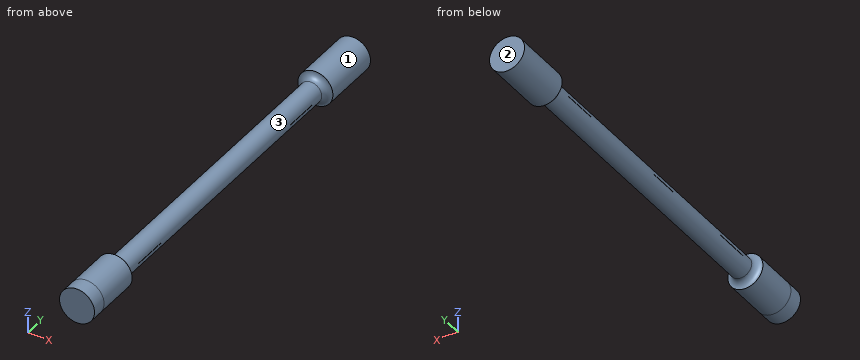
from build123d import *

# Parameters (mm, degrees)
SKETCH1_R               = 21.39
BOSS_EXTRUDE1_DEPTH     = 630
SKETCH2_R               = 35
BOSS_EXTRUDE2_DEPTH     = 88.02
BOSS_EXTRUDE3_START     = 88.02
SKETCH3_R               = 35
BOSS_EXTRUDE3_DEPTH     = 88.02
FILLET3_R               = 13.575
MOVE_FACE1_BY           = 30
MOVE_FACE2_BY           = 30
CUT_EXTRUDE1_DEPTH      = 750.655867982
CUT_EXTRUDE1_DEPTH_BACK = 750.655867982
CUT_EXTRUDE2_START      = -21.390000045
CUT_EXTRUDE2_DEPTH      = 21.390000045


# Read off the part's stored shape, not the designer's step: Cut-Extrude2
with BuildPart() as part:
    # Sketch1 → Boss-Extrude1 (new body)
    with BuildSketch(Plane(origin=(0, 0, 0), x_dir=(1, 0, 0), z_dir=(0, 1, 0))):
        with Locations(Location((0, 0, 0), (0, 0, 270))):
            Circle(SKETCH1_R)
    extrude(amount=BOSS_EXTRUDE1_DEPTH)

    # Sketch2 → Boss-Extrude2 (add)
    with BuildSketch(Plane(origin=(0, 630, 0), x_dir=(1, 0, 0), z_dir=(0, 1, 0))):
        with Locations(Location((0, 0, 0), (0, 0, 270))):
            Circle(SKETCH2_R)
    extrude(amount=BOSS_EXTRUDE2_DEPTH)

    # Sketch3 → Boss-Extrude3 (add)
    with BuildSketch(Plane.XZ.offset(BOSS_EXTRUDE3_START)):
        with Locations(Location((0, 0, 0), (0, 0, 90))):
            Circle(SKETCH3_R)
    extrude(amount=-BOSS_EXTRUDE3_DEPTH)

    # Fillet3
    fillet3_edges = [part.edges().sort_by_distance(p)[0] for p in [
        (0, 630, -21.39),
        (0, 0, -21.39),
    ]]
    fillet(fillet3_edges, radius=FILLET3_R)

    # Move Face1: a face moved outward by 30.0
    extrude(part.faces().sort_by_distance((0, 718.02, 0))[0], amount=MOVE_FACE1_BY, dir=(0, 1, 0))

    # Move Face2: a face moved outward by 30.0
    extrude(part.faces().sort_by_distance((0, -88.02, 0))[0], amount=MOVE_FACE2_BY, dir=(0, -1, 0))

    # Sketch4 → Cut-Extrude1 (cut, two sides: drawn at the far end of the back side and taken through both)
    with BuildSketch(Plane(origin=(0, 0, 0), x_dir=(0, 0, -1), z_dir=(1, 0, 0)).offset(-CUT_EXTRUDE1_DEPTH_BACK)):
        with BuildLine():
            Line((-0.43, 588.175), (-0.43, 518.175))
            ThreePointArc((-0.43, 518.175), (0, 517.745), (0.43, 518.175))
            Line((0.43, 518.175), (0.43, 588.175))
            ThreePointArc((0.43, 588.175), (0, 588.605), (-0.43, 588.175))
        make_face()
        with BuildLine():
            Line((-0.43, 111.71612329), (-0.43, 41.71612329))
            ThreePointArc((-0.43, 41.71612329), (0, 41.28612329), (0.43, 41.71612329))
            Line((0.43, 41.71612329), (0.43, 111.71612329))
            ThreePointArc((0.43, 111.71612329), (0, 112.14612329), (-0.43, 111.71612329))
        make_face()
    extrude(amount=CUT_EXTRUDE1_DEPTH + CUT_EXTRUDE1_DEPTH_BACK, mode=Mode.SUBTRACT)

    # Cut-Extrude2 outline → Cut-Extrude2 (cut)
    with BuildSketch(Plane(origin=(0, 0, 0), x_dir=(0, 0, -1), z_dir=(1, 0, 0)).offset(CUT_EXTRUDE2_START)):
        with BuildLine():
            ThreePointArc((-0.43, 260.7089), (0, 260.2789), (0.43, 260.7089))
            Line((0.43, 260.7089), (0.43, 320.7089))
            ThreePointArc((0.43, 320.7089), (0, 321.1389), (-0.43, 320.7089))
            Line((-0.43, 320.7089), (-0.43, 260.7089))
        make_face()
    extrude(amount=CUT_EXTRUDE2_DEPTH, mode=Mode.SUBTRACT)


solid = part.part
Can you work these out from the model? Positions are in its coordinate system, mm. Face numbers are marked on the shaded views. Give positions to 0.01 mm unless a question says otherwise; leave off trailing zeros. Loops run counter-clockwise (first coordinate to the right, second up) from the corner with the lowest first, then second, coordinate; pieces in that order, holes last. Notation, with made-up numbers: (19, -10.5) -> (51, -10.5) arc R18 ccw to (51, 20.5) -> close; hole circle Ø4 at (24.5, 14). An arc over 180 degrees is marked (long way). Write item = value, one per line.
1) Suppose I cut it at B-B on y = 419. Write out the boundary of the cut face in (x, z).
Check result:
outline = circle Ø42.78 at (0, 0)
2) Thinking about a two-plate mould opening in Y: for the marked faces 1, 2 and 3, which applies, released by +Y, released by -Y, zero draft, split by the parting line, or undercut?
Check result:
face_1 = zero draft
face_2 = released by +Y
face_3 = undercut
3) Suppose I cut it at C-C on x = -10.5. Give the number of separate pieces and of enclosed holes in the cut face, then the cut area to 3 significant figures.
Check result:
separate_pieces = 1
enclosed_holes = 3
area = 39,200 mm2
4) I need wall thicknesses on L1, parallel to Y at x = -18, z = -29; L2, parallel to Y at x = -6, z = 25; L3, parallel to X at y = 302, z = 2.5. Which ranges of each line are inside material? Lowest first, please. Write a range as from..to.
Check result:
L1 = -118.02..0.03, 629.97..748.02
L2 = -118.02..3.64, 626.36..748.02
L3 = -21.24..21.24
5) Will these pins go through, and if not, where does the flat tip stop? pin 1 (3 mm diameter, centred on y = 445.5, z = -1.5, fed in from -X); pin 2 (1 mm diameter, centred on y = 268.5, z = -7.5, fed in from -X); pin 3 (2 mm diameter, centred on x = 8.5, y = 24.5, fed in from -Z).
Check result:
pin_1 = -21.39
pin_2 = -20.21
pin_3 = -20.03
